Autodesk Inventor part; units mm, degrees
ref_plane "YZ Plane" through (0, 0, 0) normal (1, 0, 0) x (0, 1, 0)
ref_plane "XZ Plane" through (0, 0, 0) normal (0, 1, 0) x (-1, 0, 0)
ref_plane "XY Plane" through (0, 0, 0) normal (0, 0, 1) x (1, 0, 0)
sketch "Эскиз1" plane through (0, 0, 0) normal (0, 1, 0) x (-1, 0, 0)
  line L0 (-29.25, 11) -> (29.25, 11)
  line L1 (29.25, 11) -> (29.25, -11)
  line L2 (29.25, -11) -> (-29.25, -11)
  line L3 (-29.25, -11) -> (-29.25, 11)
  line L4 (-29.25, 11) -> (29.25, -11) construction
  line L5 (29.25, 11) -> (-29.25, -11) construction
  line L6 (-29.25, 11) -> (-4.25, 11)
  line L7 (-4.25, 11) -> (-4.25, 23)
  line L8 (-4.25, 23) -> (-29.25, 23)
  line L9 (-29.25, 23) -> (-29.25, 11)
  point P0 (0, 0)
  dimension "d0" = 22
  dimension "d1" = 58.5
  dimension "d8" = 34
  dimension "d9" = 25
extrude "Выдавливание1" add sketch "Эскиз1" along normal blind 3
sketch "Эскиз2" plane through (-29.25, 0, -11) normal (-1, 0, 0) x (0, 0, 1)
  line L0 (0, 0) -> (22, 0)
  line L1 (22, 0) -> (22, 3)
  line L2 (0, 3) -> (22, 3)
  line L3 (0, 0) -> (0, 3)
  line L4 (0, 3) -> (22, 3)
  line L5 (22, 3) -> (0, 3)
  line L6 (0, 3) -> (0, -25)
  line L7 (0, -25) -> (22, -25)
  line L8 (22, -25) -> (22, 3)
  line L9 (22, -25) -> (22, -3.9)
  line L10 (22, -3.9) -> (34, -3.9)
  line L11 (34, -3.9) -> (34, -25)
  line L12 (34, -25) -> (22, -25)
  point P0 (11, 0)
  point P1 (22, 0)
  point P2 (22, 3)
  dimension "d4" = 28
  dimension "d7" = 22
  dimension "d13" = 34
  dimension "d14" = 21.1
extrude "Выдавливание2" add sketch "Эскиз2" along normal blind 3
sketch "Эскиз3" plane through (4.25, 0, 23) normal (0, 0, 1) x (1, 0, 0)
  line L0 (0, 0) -> (25, 0)
  line L1 (25, 0) -> (25, 3)
  line L2 (0, 3) -> (25, 3)
  line L3 (0, 0) -> (0, 3)
  line L4 (25, 0) -> (25, 3)
  line L5 (0, 0) -> (0, 3)
  line L6 (25, 3) -> (0, 3)
  line L7 (0, 3) -> (0, -25)
  line L8 (0, -25) -> (25, -25)
  line L9 (25, -25) -> (25, 3)
  point P0 (-4.25, 0)
  dimension "d10" = 28
extrude "Выдавливание3" add sketch "Эскиз3" along normal blind 3
sketch "Эскиз4" plane through (-29.25, -25, 23) normal (0, 0, 1) x (1, 0, 0)
  line L0 (0, 0) -> (0, 21.1)
  line L1 (0, 21.1) -> (-3, 21.1)
  line L2 (-3, 0) -> (-3, 21.1)
  line L3 (0, 0) -> (-3, 0)
  line L4 (-3, 0) -> (-3, 21.1)
  line L5 (-3, 21.1) -> (25, 21.1)
  line L6 (25, 21.1) -> (25, 0)
  line L7 (25, 0) -> (-3, 0)
  point P0 (29.25, 25)
  dimension "d15" = 28
extrude "Выдавливание4" add sketch "Эскиз4" along normal blind 3
fillet "Сопряжение1" radius 2 4 edges at (-29.25, 0, 0) (-32.25, 3, 0) (16.75, 3, 26) (16.75, 0, 23)
fillet "Сопряжение1" radius 4 10 edges at (-32.25, -14.45, 26) (-29.25, -14.45, 23) (-4.25, -3.9, 24.5) (-4.25, -25, 24.5) (-30.75, -3.9, 11) (4.25, 1.5, 11) (4.25, -25, 24.5) (29.25, -25, 24.5) (-30.75, -25, -11) (29.25, 1.5, -11)
sketch "Эскиз5" plane through (4.25, 0, 26) normal (0, 0, 1) x (1, 0, 0)
  circle A0 centre (6, -14.45) radius 1.8
  circle A1 centre (19, -14.45) radius 1.8
  arc A2 (21, -25) -> (25, -21) centre (21, -21) ccw
  line L0 (25, -21) -> (25, 1)
  line L1 (0, 1) -> (25, 1)
  line L2 (0, 1) -> (0, -21)
  arc A3 (0, -21) -> (4, -25) centre (4, -21) ccw
  line L3 (4, -25) -> (21, -25)
  line L4 (4, -25) -> (21, -25) construction
  line L5 (12.5, -25) -> (12.5, 1) construction
  line L6 (6, -14.45) -> (19, -14.45) construction
  line L7 (0, 0) -> (25, 0) construction
  arc A4 (-12.5, -25) -> (-8.5, -21) centre (-12.5, -21) ccw
  line L8 (-8.5, -21) -> (-8.5, -7.9)
  arc A5 (-8.5, -7.9) -> (-12.5, -3.9) centre (-12.5, -7.9) ccw
  line L9 (-12.5, -3.9) -> (-32.5, -3.9)
  line L10 (-32.5, -25) -> (-32.5, -3.9)
  line L11 (-32.5, -25) -> (-12.5, -25)
  line L12 (-36.5, -3.9) -> (-36.5, -25)
  circle A6 centre (-19.5, -19.45) radius 2.2361
  circle A7 centre (-19.5, -9.45) radius 2.6907
  line L13 (-19.5, -19.45) -> (-19.5, -9.45) construction
  line L14 (-19.5, -14.45) -> (-4.25, -14.45) construction
  point P0 (-4.25, 0)
  dimension "d21" = 3.6
  dimension "d22" = 3.6
  dimension "d23" = 13
  dimension "d33" = 13
  dimension "d34" = 10
  dimension "d35" = 21.1
  dimension "d36" = 10.55
hole "Отверстие1" at (10.25, -14.45, 26) at (23.25, -14.45, 26) at (-15.25, -9.45, 26) at (-15.25, -19.45, 26) direction (0, 0, -1) diameter 3.6 depth 5 countersink diameter 6.6 countersink angle 90
sketch "Эскиз6" plane through (-32.25, 0, -11) normal (-1, 0, 0) x (0, 0, 1)
  line L0 (32, 0) -> (4, 0) construction
  line L1 (22, 0) -> (0, 0) construction
  line L2 (0, 0) -> (0, -25) construction
  line L3 (0, -25) -> (22, -25) construction
  line L4 (22, -25) -> (22, 0) construction
  arc A0 (0, -21) -> (4, -25) centre (4, -21) ccw construction
  line L5 (4, -25) -> (33, -25) construction
  line L6 (33, -3.9) -> (33, -25) construction
  line L7 (26, -3.9) -> (33, -3.9) construction
  arc A1 (22, 0.1) -> (26, -3.9) centre (26, 0.1) ccw construction
  line L8 (22, 0.1) -> (22, 1) construction
  line L9 (0, 1) -> (22, 1) construction
  line L10 (0, 1) -> (0, -21) construction
  circle A2 centre (11, -12.5) radius 2.7933
  arc A3 (22, 0.1) -> (26, -3.9) centre (26, 0.1) ccw construction
  line L11 (22, 0.1) -> (0, -25) construction
  line L12 (0, 0) -> (0, -2) construction
  line L13 (22, -25) -> (0, 0) construction
  point P0 (11, 0)
hole "Отверстие2" at (-32.25, -12.5, 0) direction (1, 0, 0) diameter 3.6 depth 6 countersink diameter 6.6 countersink angle 90
sketch "Эскиз7" plane through (0, 3, 0) normal (0, 1, 0) x (1, 0, 0)
  arc A0 (29.25, 7) -> (25.25, 11) centre (25.25, 7) ccw construction
  line L0 (25.25, 11) -> (-30.25, 11) construction
  line L1 (-30.25, -11) -> (-30.25, 11) construction
  line L2 (0.25, -11) -> (-30.25, -11) construction
  arc A1 (4.25, -15) -> (0.25, -11) centre (0.25, -15) ccw construction
  line L3 (4.25, -15) -> (4.25, -24) construction
  line L4 (29.25, -24) -> (4.25, -24) construction
  line L5 (29.25, 7) -> (29.25, -24) construction
  line L6 (29.25, -11) -> (29.25, 11) construction
  line L7 (29.25, 11) -> (-29.25, 11) construction
  line L8 (29.25, 7) -> (29.25, -24) construction
  line L9 (-29.2407, 0) -> (29.25, 0) construction
  line L10 (29.25, -21) -> (29.25, 7) construction
  line L11 (-29.25, -11.5956) -> (-29.25, 11) construction
  line L12 (-29.25, -11) -> (-29.25, 11) construction
  line L13 (-29.25, -11) -> (29.25, -11) construction
  circle A2 centre (-15, 0) radius 3.1623 construction
  circle A3 centre (15, 0) radius 5 construction
  line L14 (0, 0) -> (0, 6.5971) construction
  point P0 (-32.25, -11)
  point P1 (-29.25, 0)
  dimension "d44" = 30
hole "Отверстие3" at (-15, 3, 0) at (15, 3, 0) direction (0, -1, 0) diameter 3.6 depth 6 countersink diameter 6.6 countersink angle 90
equation "\"d36\" = 0.5 * d35"
properties part number "кронштейн"
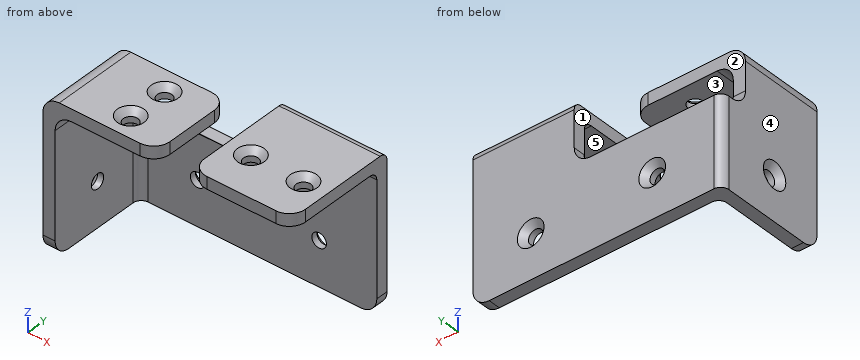
Geometry check sheet. Reference: the model listing, model coordinates, mm. Face numbers are marked on the shaded views. A direction names the side the tool comes from. Round coordinates to 2 decimals unless told otherwise and drop trailing zeros. Write each loop counter-clockwise with the first axis right and the second up, starting at its lowest first coordinate (ties: lowest second). Pieces come first, ordered by that corner, then holes.
Item 1: Section check C-C (z = 0). Record the boundary of the cut face in (x, y).
Determined:
outline: (-32.25, -25) - (-29.25, -25) - (-29.25, -14.3) - (-30.75, -14.3) - (-32.25, -15.8) - close; (-32.25, -9.2) - (-30.75, -10.7) - (-29.25, -10.7) - (-29.25, -2) arc R2 cw to (-27.25, 0) - (-16.8, 0) - (-16.8, 1.5) - (-18.3, 3) - (-30.25, 3) arc R2 ccw to (-32.25, 1) - close; (-13.2, 0) - (13.2, 0) - (13.2, 1.5) - (11.7, 3) - (-11.7, 3) - (-13.2, 1.5) - close; (16.8, 0) - (29.25, 0) - (29.25, 3) - (18.3, 3) - (16.8, 1.5) - close
Item 2: Section check A-A (x = 10.25). Record the boundary of the cut face in (y, z), plus the area to 3 significant figures.
Determined:
outline: (-25, 23) - (-16.25, 23) - (-16.25, 24.5) - (-17.75, 26) - (-25, 26) - close; (-12.65, 23) - (-2, 23) arc R2 cw to (0, 21) - (0, -11) - (3, -11) - (3, 24) arc R2 ccw to (1, 26) - (-11.15, 26) - (-12.65, 24.5) - close
area: 173 mm2
Item 3: Access from +Z, -Z, +X, -X, +Y, -Y to the whole of each face (thin tool, end or side, straight path). Record for the marked faces 1, 2, 3, 4 and 5.
Determined:
face 1: +Z, +Y, -Y
face 2: +Z, -X, +Y
face 3: -Z, +X, +Y, -Y
face 4: +Z, -Z, -X, +Y, -Y
face 5: -Z, +X, -Y
Item 4: Material ranges on line 1 along Y through (x, z) = (-15.25, 24.05); line 2 along X through (y, z) = (0.55, 0); line 3 along Y through (x, z) = (10.25, 24.25), recorded low to high.
Determined:
line 1: y = -25 to -21.25, -17.65 to -11.25, -7.65 to -3.9
line 2: x = -32.25 to -16.8, -13.2 to 13.2, 16.8 to 29.25
line 3: y = -25 to -16.25, -12.65 to 2.98
Item 5: Go/stop test with flat-tipped pins: pin 1 Ø9 at (x, z) = (-25.5, 23) entering from +Y; pin 2 Ø4.5 at (x, y) = (10.25, -14.45) entering from -Z; pin 3 Ø1.4 at (x, y) = (-10.5, 1) entering from +Z; pin 4 Ø2 at (x, z) = (-15, 0) entering from -Y. Record where each tip stops, or that it passes through.
Determined:
pin 1: stops at y = -3.9
pin 2: stops at z = 23
pin 3: stops at z = 11
pin 4: passes through
Item 6: Section check D-D (x = -11). Record the boundary of the cut face in (y, z), plus the area to 3 significant figures.
Determined:
outline: (-25, 23) - (-3.9, 23) - (-3.9, 26) - (-25, 26) - close; (0, -11) - (3, -11) - (3, 11) - (0.1, 11) arc R4 cw to (0, 11) - close
area: 129 mm2
Item 7: Section check B-B (y = -19.45). Record the boundary of the cut face in (x, z), plus the area to 3 significant figures.
Determined:
outline: (-32.25, -11) - (-29.25, -11) - (-29.25, 19) arc R4 cw to (-25.25, 23) - (-17.05, 23) - (-17.05, 24.5) - (-18.55, 26) - (-28.25, 26) arc R4 ccw to (-32.25, 22) - close; (-13.45, 23) - (-4.25, 23) - (-4.25, 26) - (-11.95, 26) - (-13.45, 24.5) - close; (4.25, 23) - (29.25, 23) - (29.25, 26) - (4.25, 26) - close
area: 248 mm2
